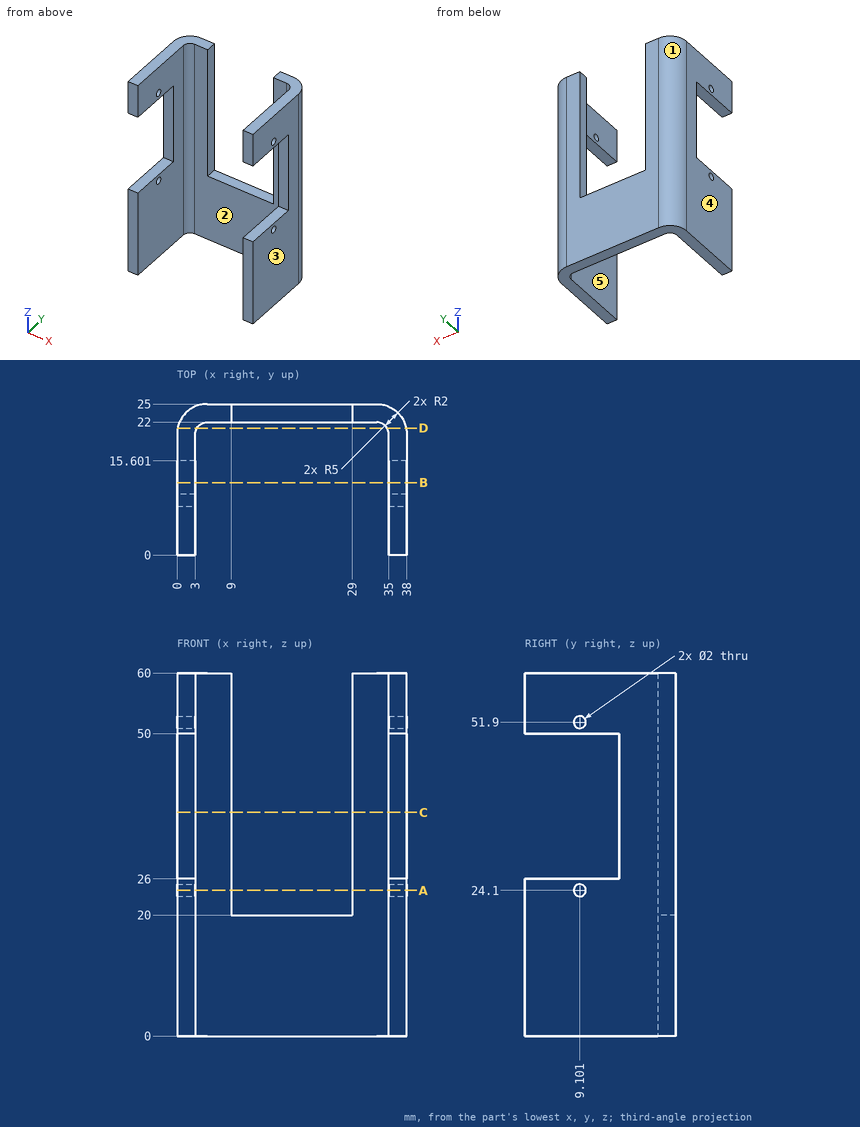
Geometry check sheet. Reference: drawing and pictorial views, mm from the part's lowest x, y, z. A direction names the side the tool comes from. Give positions to 0.01 mm unless a question says otherwise; leave off trailing zeros. Order: outer loops, then holes, each group sorted by start corner. A loop starts at its lowest first (then second) coordinate and runs counter-clockwise, first axis right, second up. Notation, with made-up numbers: M 12.25,36.25 L 69.25,36.25 A29 ccw 69.25,63.25 Z; hole C 51.25,-11 d7. An arc over 180 degrees is marked long. Answer in a Markdown table with one row per item. Add a question column.
Item 1: Tool access check on the marked faces 1 and 2. Record the directions out of +Z, -Z, +X, -X, +Y, -Y that give a thin tool (end or side, any length) a straight path to the whole face; none if there is none.
Item 2: Section check A-A, the plane z = 24.1. Enter the section's corners in (x, y), and give its area (3 significant figures).
Item 3: Mould release check, pull along X, two halves, no side actions. Record for the marked faces 3, 4 and 5: released by +X, released by -X, zero draft, split by the parting line, or undercut.
Item 4: Scan lines: probe 1 along X at (y, z) = (19.25, 32.5); probe 2 along Z at (x, y) = (2.5, 9.75); probe 3 along Z at (x, y) = (35.5, 14). Record each from-to range of solid material in increasing order. Write a range as from..to.
Item 5: Section check D-D, the plane y = 21. Enter the section's corners in (x, z), and give its area (3 significant figures).
Item 6: Section check B-B, the plane y = 12. Enter the section's corners in (x, z), and give its area (3 significant figures).
Item 7: Gauge pin test, flat ends, axial feed: pin 1 (5 mm diameter, centred on x = 6.5, z = 47, fed in from -Y); pin 2 (3.5 mm diameter, centred on x = 21, y = 24, fed in from +Z); pin 3 (2.5 mm diameter, centred on y = 23, z = 46.5, fed in from -X). Record the tip position at first contact, or that the pin passes through.
Item 8: Section check C-C, the plane z = 37. Enter the section's corners in (x, y).
Filled sheet:
| question | item | result |
|---|---|---|
| 1 | face 1 | +Z, -Z, -X, +Y |
| 1 | face 2 | +Z, -Z, -Y |
| 2 | outline | M 0,0 L 3,0 L 3,8.1 L 0,8.1 Z; M 0,10.1 L 3,10.1 L 3,20 A2 cw 5,22 L 9,22 L 9,25 L 5,25 A5 ccw 0,20 Z; M 29,22 L 33,22 A2 cw 35,20 L 35,10.1 L 38,10.1 L 38,20 A5 ccw 33,25 L 29,25 Z; M 35,0 L 38,0 L 38,8.1 L 35,8.1 Z |
| 2 | area | 165 mm^2 |
| 3 | face 3 | released by +X |
| 3 | face 4 | released by -X |
| 3 | face 5 | undercut |
| 4 | probe 1 | x = 0..3, 35..38 |
| 4 | probe 2 | z = 0..23.34, 24.86..26, 50..51.14, 52.66..60 |
| 4 | probe 3 | z = 0..26, 50..60 |
| 5 | outline | M 0.1,0 L 3.27,0 L 3.27,60 L 0.1,60 Z; M 34.73,0 L 37.9,0 L 37.9,60 L 34.73,60 Z |
| 5 | area | 380 mm^2 |
| 6 | outline | M 0,0 L 3,0 L 3,26 L 0,26 Z; M 0,50 L 3,50 L 3,60 L 0,60 Z; M 35,0 L 38,0 L 38,26 L 35,26 Z; M 35,50 L 38,50 L 38,60 L 35,60 Z |
| 6 | area | 216 mm^2 |
| 7 | pin 1 | stops at y = 21.73 |
| 7 | pin 2 | stops at z = 20 |
| 7 | pin 3 | stops at x = 0.32 |
| 8 | outline | M 0,15.6 L 3,15.6 L 3,20 A2 cw 5,22 L 9,22 L 9,25 L 5,25 A5 ccw 0,20 Z; M 29,22 L 33,22 A2 cw 35,20 L 35,15.6 L 38,15.6 L 38,20 A5 ccw 33,25 L 29,25 Z |
